Could you check a few things on this model? Use its own coordinates, in mm. Round coordinates to 2 decimals unless told otherwise and drop trailing zeros. Loops run counter-clockwise (first coordinate to the right, second up) from the corner with the lowest first, then second, coordinate; pieces in that order, holes last. Notation, with made-up numbers: M 18.25,-2 L 22.25,-2 A11 ccw 22.25,8 Z; hole C 9.25,67 d7. An arc over 180 degrees is marked long. Answer in a Markdown table with one row per item.
```python
from build123d import *

# Parameters (mm, degrees)
SKETCH_1_W                         = 2.79
SKETCH_1_H                         = 5
EXTRUDE_1_DEPTH                    = 8.4
SKETCH_2_W                         = 1
SKETCH_2_H                         = 1
CUT_EXTRUDE_1_DEPTH                = 8
CHAMFER_1_SIZE                     = 0.2
SKETCH_3_W                         = 0.64
SKETCH_3_H                         = 0.64
EXTRUDE_2_DEPTH                    = 2.29
CHAMFER_2_SIZE                     = 0.2
PATTERN_LINEAR_1_COUNT             = 4
PATTERN_LINEAR_1_PITCH             = 2.54
CHAMFER_1_OF_PATTERN_LINEAR_1_SIZE = 0.2
CHAMFER_2_OF_PATTERN_LINEAR_1_SIZE = 0.2


with BuildPart() as part:
    # Эскиз1 → Бобышка-Вытянуть1 (new body)
    with BuildSketch(Plane(origin=(0, 0, 0), x_dir=(1, 0, 0), z_dir=(0, 1, 0))):
        Rectangle(SKETCH_1_W, SKETCH_1_H)
    extrude_1 = extrude(amount=EXTRUDE_1_DEPTH)

    # Эскиз2 → Вырез-Вытянуть1 (cut)
    with BuildSketch(Plane(origin=(0, 8.4, 0), x_dir=(1, 0, 0), z_dir=(0, 1, 0))):
        with Locations((0, 1.27)):
            Rectangle(SKETCH_2_W, SKETCH_2_H)
        with Locations((0, -1.27)):
            Rectangle(SKETCH_2_W, SKETCH_2_H)
    cut_extrude_1 = extrude(amount=-CUT_EXTRUDE_1_DEPTH, mode=Mode.SUBTRACT)

    # Фаска1
    chamfer_1_edges = [part.edges().sort_by_distance(p)[0] for p in [
        (0.5, 8.4, -1.27),
        (0, 8.4, -1.77),
        (-0.5, 8.4, -1.27),
        (0, 8.4, -0.77),
        (0, 8.4, 1.77),
        (0.5, 8.4, 1.27),
        (0, 8.4, 0.77),
        (-0.5, 8.4, 1.27),
    ]]
    chamfer(chamfer_1_edges, length=CHAMFER_1_SIZE)

    # Эскиз3 → Бобышка-Вытянуть2 (add)
    with BuildSketch(Plane(origin=(0, 0, 0), x_dir=(-1, 0, 0), z_dir=(0, -1, 0))):
        with Locations((0, 1.27)):
            Rectangle(SKETCH_3_W, SKETCH_3_H)
        with Locations((0, -1.27)):
            Rectangle(SKETCH_3_W, SKETCH_3_H)
    extrude_2 = extrude(amount=EXTRUDE_2_DEPTH)

    # Фаска2
    chamfer_2_edges = [part.edges().sort_by_distance(p)[0] for p in [
        (0.32, -2.29, -1.27),
        (0, -2.29, -0.95),
        (-0.32, -2.29, -1.27),
        (0, -2.29, -1.59),
        (-0.32, -2.29, 1.27),
        (0, -2.29, 0.95),
        (0.32, -2.29, 1.27),
        (0, -2.29, 1.59),
    ]]
    chamfer(chamfer_2_edges, length=CHAMFER_2_SIZE)

    # Линейный массив1: Бобышка-Вытянуть1, Вырез-Вытянуть1, Бобышка-Вытянуть2 ×4
    with Locations(*[(i * PATTERN_LINEAR_1_PITCH, 0, 0) for i in range(1, PATTERN_LINEAR_1_COUNT)]):
        add(extrude_1)
        add(cut_extrude_1, mode=Mode.SUBTRACT)
        add(extrude_2)

    # Фаска1 of Линейный массив1
    chamfer_1_of_pattern_linear_1_edges = [part.edges().sort_by_distance(p)[0] for p in [
        (3.04, 8.4, -1.27),
        (2.54, 8.4, -1.77),
        (2.04, 8.4, -1.27),
        (2.54, 8.4, -0.77),
        (2.54, 8.4, 1.77),
        (3.04, 8.4, 1.27),
        (2.54, 8.4, 0.77),
        (2.04, 8.4, 1.27),
        (5.58, 8.4, -1.27),
        (5.08, 8.4, -1.77),
        (4.58, 8.4, -1.27),
        (5.08, 8.4, -0.77),
        (5.08, 8.4, 1.77),
        (5.58, 8.4, 1.27),
        (5.08, 8.4, 0.77),
        (4.58, 8.4, 1.27),
        (8.12, 8.4, -1.27),
        (7.62, 8.4, -1.77),
        (7.12, 8.4, -1.27),
        (7.62, 8.4, -0.77),
        (7.62, 8.4, 1.77),
        (8.12, 8.4, 1.27),
        (7.62, 8.4, 0.77),
        (7.12, 8.4, 1.27),
    ]]
    chamfer(chamfer_1_of_pattern_linear_1_edges, length=CHAMFER_1_OF_PATTERN_LINEAR_1_SIZE)

    # Фаска2 of Линейный массив1
    chamfer_2_of_pattern_linear_1_edges = [part.edges().sort_by_distance(p)[0] for p in [
        (2.86, -2.29, -1.27),
        (2.54, -2.29, -0.95),
        (2.22, -2.29, -1.27),
        (2.54, -2.29, -1.59),
        (2.22, -2.29, 1.27),
        (2.54, -2.29, 0.95),
        (2.86, -2.29, 1.27),
        (2.54, -2.29, 1.59),
        (5.4, -2.29, -1.27),
        (5.08, -2.29, -0.95),
        (4.76, -2.29, -1.27),
        (5.08, -2.29, -1.59),
        (4.76, -2.29, 1.27),
        (5.08, -2.29, 0.95),
        (5.4, -2.29, 1.27),
        (5.08, -2.29, 1.59),
        (7.94, -2.29, -1.27),
        (7.62, -2.29, -0.95),
        (7.3, -2.29, -1.27),
        (7.62, -2.29, -1.59),
        (7.3, -2.29, 1.27),
        (7.62, -2.29, 0.95),
        (7.94, -2.29, 1.27),
        (7.62, -2.29, 1.59),
    ]]
    chamfer(chamfer_2_of_pattern_linear_1_edges, length=CHAMFER_2_OF_PATTERN_LINEAR_1_SIZE)


solid = part.part
```
1) I need wall thicknesses on line 1 (Z direction, x = 2.25, y = 2.5); line 2 (X direction, y = 5.5, z = -1.4) (3 decimals); line 3 (Z direction, x = 5, y = -0.5). Which ranges of each line are inside material? Lowest first, please.
Computed:
| item | result |
|---|---|
| line 1 | z = -2.5 to -1.77, -0.77 to 0.77, 1.77 to 2.5 |
| line 2 | x = -1.395 to -0.5, 0.5 to 2.04, 3.04 to 4.58, 5.58 to 7.12, 8.12 to 9.015 |
| line 3 | z = -1.59 to -0.95, 0.95 to 1.59 |
2) If we mould it in two halves opening along X, with no side actions, what happens to faces 1 (the face through (4, 4, -2.5)), 2 (the face through (9.015, 4, 0)), 3 (the face through (2.5, 4.4, -0.77)), 4 (the face through (-0.5, 4, -1))? For each: released by +X, released by -X, zero draft, split by the parting line, or undercut.
Computed:
| item | result |
|---|---|
| face 1 | zero draft |
| face 2 | released by +X |
| face 3 | undercut |
| face 4 | undercut |
3) I want a section at A-A, the plane y = 2.5. State how many separate pieces and enclosed holes the cut face has, plus the area to 4 significant figures.
Computed:
| item | result |
|---|---|
| separate pieces | 1 |
| enclosed holes | 8 |
| area | 44.05 mm² |
4) Will these pins go through, and if not, where does the flat tip stop? P1, Ø0.7, axis at y = -0.5, z = -1.5, coming from the +X side; P2, Ø0.5, axis at y = -1, z = 1.5, coming from the -X side; P3, Ø0.5, axis at x = 7.5, y = -1, coming from the +Z side.
Computed:
| item | result |
|---|---|
| P1 | stops at x = 7.94 |
| P2 | stops at x = -0.32 |
| P3 | stops at z = 1.59 |
5) I want a section at B-B, the plane z = -0.1. Please give me the cut outline in (x, y) (3 decimals).
Computed:
| item | result |
|---|---|
| outline | M -1.395,0 L 9.015,0 L 9.015,8.4 L -1.395,8.4 Z |
6) I want a section at C-C, the plane x = 6.5. Please give me the cut outline in (y, z).
Computed:
| item | result |
|---|---|
| outline | M 0,-2.5 L 8.4,-2.5 L 8.4,2.5 L 0,2.5 Z |
